Build history of the part. All positions in model axes, mm. A direction names the side the tool comes from. Coordinates: 2 decimals unless noted, no trailing zeros. Order: outer loops, then holes, each group sorted by start corner. A loop starts at its lowest first (then second) coordinate and runs counter-clockwise, first axis right, second up. Notation, with made-up numbers: (68, 67) - (120, 67) arc R24 ccw to (120, 99) - close; hole circle Ø5 at (77, -34). An arc over 180 degrees is marked (long way). Return JSON: item names as keys, results as strings.
Autodesk Inventor part; units mm, degrees
ref_plane "YZ Plane" through (0, 0, 0) normal (1, 0, 0) x (0, 1, 0)
ref_plane "XZ Plane" through (0, 0, 0) normal (0, 1, 0) x (-1, 0, 0)
ref_plane "XY Plane" through (0, 0, 0) normal (0, 0, 1) x (1, 0, 0)
sketch "Sketch1" plane through (0, 0, 0) normal (0, 0, 1) x (1, 0, 0)
  line L0 (0, -5.3) -> (0, 21.3)
  line L1 (0, 17.5) -> (-12.5, 17.5)
  line L2 (-12.5, 17.5) -> (-12.5, 1.5)
  line L3 (-12.5, 1.5) -> (-19.75, 1.5)
  line L4 (-19.75, 1.5) -> (-19.75, -1.5)
  line L5 (-19.75, -1.5) -> (-13.5, -1.5)
  line L6 (-13.5, -1.5) -> (-13.5, -1)
  line L7 (-13.5, -1) -> (0, -1)
  point P0 (0, 0)
  point P1 (-19.75, 0)
  dimension "d0" = 39.5
  dimension "d1" = 25
  dimension "d2" = 3
  dimension "d3" = 16
  dimension "d4" = 27
  dimension "d5" = 0.5
revolve "Revolution1" add sketch "Sketch1" angle 360 about axis through (0, -10, 0) along (0, 1, 0)
sketch "Sketch2" plane through (0, -1.5, 0) normal (0, -1, 0) x (1, 0, 0)
  point P0 (0, 0)
  point P1 (0, 0)
hole "Hole1" at (0, -1.5, 0) direction (0, 1, 0) diameter 8.376 depth 15 tip angle 118
chamfer "Chamfer1" distance 3 angle 45 1 edges at (12.5, 1.5, 0)
chamfer "Chamfer2" distance 0.8 angle 45 2 edges at (19.75, 1.5, 0) (19.75, -1.5, 0)
chamfer "Chamfer3" distance 3 angle 45 1 edges at (12.5, 17.5, 0)
properties part number "Base Plate" material "Steel, Mild"
1. Tool access for faces 1 (the cylindrical face through (-11.923, 9.43, -3.755)), 2 (the flat face through (3.2, -1, 3.2)), 3 (the flat face through (4.5, -1.5, 12.9)): list every direction of +Z, -Z, +X, -X, +Y, -Y with a clear straight run to the whole face (end or side of a thin tool).
Check values:
{"face 1": "+Y", "face 2": "-Y", "face 3": "+Z, -Z, +X, -X, -Y"}
2. Cut at A-A on y = 11.25. Give the cut face in (x, z).
Check values:
{"outline": "circle Ø25 at (0, 0); hole circle Ø8.38 at (0, 0)"}
3. Mould opens along X. For faces 4 (the conical face through (-12.102, 4.312, -3.811)), 5 (the cylindrical face through (-2.83, 6.352, 3.087)), 6 (the flat face through (16, 1.5, 0)) say: pulls with the +X half, pulls with the -X half, needs draft (parallel to the pull), parting line crosses it, or undercut.
Check values:
{"face 4": "parting line crosses it", "face 5": "undercut", "face 6": "needs draft"}
4. Drop flat-ended pins along their axis: pin 1 (19 mm diameter, centred on x = 9.5, z = -8.5, fed in from +Y); pin 2 (1.5 mm diameter, centred on x = 12.5, y = 1, fed in from -Z); pin 3 (5 mm diameter, centred on x = -2, z = -4.5, fed in from -Y); pin 4 (10 mm diameter, centred on x = 7, y = 8, fed in from +Z). Give the stop position or say it passes through.
Check values:
{"pin 1": "y = 17.5", "pin 2": "z = -15.83", "pin 3": "y = -1", "pin 4": "z = 12.64"}
5. Cut at B-B on y = 15.5. Give the cut face in (x, z), plus the area to 3 significant figures.
Check values:
{"outline": "circle Ø23 at (0, 0); hole circle Ø1.72 at (0, 0)", "area": "413 mm²"}
6. Probe L1, parallel to Y at x = 5.5, z = 1.5; L2, parallel to X at y = 4, z = 0; L3, parallel to Z at x = 0, y = 2.25. List the from-to ranges inside material, lowest first.
Check values:
{"L1": "-1 to 17.5", "L2": "-13 to -4.19, 4.19 to 13", "L3": "-14.75 to -4.19, 4.19 to 14.75"}
